Autodesk Inventor part; units mm, degrees
ref_plane "Plan YZ" through (0, 0, 0) normal (1, 0, 0) x (0, 1, 0)
ref_plane "Plan XZ" through (0, 0, 0) normal (0, 1, 0) x (-1, 0, 0)
ref_plane "Plan XY" through (0, 0, 0) normal (0, 0, 1) x (1, 0, 0)
sketch "Esquisse7" plane through (0, 0, 0) normal (0, 0, 1) x (1, 0, 0)
  line L0 (-88, -26) -> (-88, 26)
  line L1 (-88, 26) -> (-83, 26)
  line L2 (-83, 26) -> (-83, 29)
  line L3 (-83, 29) -> (-68, 29)
  line L4 (-68, 29) -> (-68, 26)
  line L5 (-68, 26) -> (-7.5, 26)
  line L6 (-7.5, 26) -> (-7.5, 29)
  line L7 (-7.5, 29) -> (7.5, 29)
  line L8 (7.5, 29) -> (7.5, 26)
  line L9 (7.5, 26) -> (68, 26)
  line L10 (68, 26) -> (68, 29)
  line L11 (68, 29) -> (83, 29)
  line L12 (83, 29) -> (83, 26)
  line L13 (83, 26) -> (88, 26)
  line L14 (88, 26) -> (88, -26)
  line L15 (88, -26) -> (83, -26)
  line L16 (83, -26) -> (83, -29)
  line L17 (83, -29) -> (68, -29)
  line L18 (68, -29) -> (68, -26)
  line L19 (7.5, -26) -> (7.5, -29)
  line L20 (7.5, -26) -> (68, -26)
  line L21 (7.5, -29) -> (-7.5, -29)
  line L22 (-7.5, -29) -> (-7.5, -26)
  line L23 (-7.5, -26) -> (-68, -26)
  line L24 (-68, -26) -> (-68, -29)
  line L25 (-68, -29) -> (-83, -29)
  line L26 (-83, -29) -> (-83, -26)
  line L27 (-83, -26) -> (-88, -26)
  line L28 (0, -40.6) -> (0, 40.6) construction
  line L29 (-123.2, 0) -> (123.2, 0) construction
  dimension "d33" = 52
  dimension "d34" = 15
  dimension "d35" = 3
  dimension "d36" = 5
  dimension "d65" = 176
extrude "Extrusion2" add sketch "Esquisse7" against normal blind 3
sketch "Esquisse8" plane through (0, 0, 0) normal (0, 0, 1) x (1, 0, 0)
  point P0 (0, 0)
  point P1 (7.5, 26)
  point P2 (-7.5, 26)
  point P3 (-83, 26)
  point P4 (-68, 26)
  point P5 (-83, -26)
  point P6 (-68, -26)
  point P7 (-7.5, -26)
  point P8 (7.5, -26)
  point P9 (68, -26)
  point P10 (83, -26)
  point P11 (68, 26)
  point P12 (83, 26)
  point P13 (83, 26)
  point P14 (68, -26)
  point P15 (83, 26)
hole "Perçage2" at (7.5, 26, 0) at (-7.5, 26, 0) at (-83, 26, 0) at (-68, 26, 0) at (-83, -26, 0) at (-68, -26, 0) at (-7.5, -26, 0) at (7.5, -26, 0) at (68, -26, 0) at (83, -26, 0) at (68, 26, 0) at (83, 26, 0) direction (0, 0, -1) diameter 1 end through all
chamfer "Chanfrein3" distance 1 angle 45 12 edges at (-83, -29, -1.5) (-68, -29, -1.5) (-83, 29, -1.5) (-68, 29, -1.5) (-7.5, 29, -1.5) (7.5, 29, -1.5) (68, 29, -1.5) (83, 29, -1.5) (68, -29, -1.5) (83, -29, -1.5) (-7.5, -29, -1.5) (7.5, -29, -1.5)
properties part number "P1704_102" material "Plastique PMMA"
Geometry: final body of the model. Coordinates: model frame, mm. A direction names the side the tool comes from. Coordinates: 2 decimals unless noted, no trailing zeros. Loops run counter-clockwise (first coordinate to the right, second up) from the corner with the lowest first, then second, coordinate; pieces in that order, holes last. Notation, with made-up numbers: (37.5, 52.5) - (43.5, 52.5) arc R11 ccw to (43.5, 62.5) - close; hole circle Ø3 at (-19.5, 76). An arc over 180 degrees is marked (long way). One line per question, with ' | ' between items. Start each with the question number.
(1) Reachability of faces 1 (the flat face through (-86, -26, -1)), 2 (the flat face through (86, -26, -1)), 3 (the flat face through (-86, 26, -1)), 4 (the flat face through (-37, -26, -1)) from +Z, -Z, +X, -X, +Y, -Y: full face, straight path, thin tool, end or side. Return the list, or none.
(2) First-contact query: pin 1 (1.6 mm diameter, centred on y = 27.5, z = -1.5, fed in from -X); pin 2 (0.9 mm diameter, centred on x = -86.5, z = -1, fed in from -Y); pin 3 (0.8 mm diameter, centred on y = 27.5, z = -1, fed in from +X). Flat tips, straight axial feed; report the tip coordinate or a pass-through.
(3) Draft query along X for faces 5 (the flat face through (0, -29, -1)), 6 (the flat face through (-88, 0, -1)), 7 (the flat face through (37, -26, -1)). Return one class per face: +X half, -X half, draft (parallel to the pull), parting line (faces both ways), or undercut.
(4) Ray query, L1, parallel to Y at x = 27, z = -1.65. Return the intervals inside material, ascending. Write a range as from..to.
(5) Cut plane A-A on x = 62. Output: boundary loops of the cut face in (y, z), and give its area (3 significant figures).
Here are the results:
1) face 1: +Z, -Z, -X, -Y | face 2: +Z, -Z, +X, -Y | face 3: +Z, -Z, -X, +Y | face 4: +Z, -Z, -Y
2) pin 1: x = -83 | pin 2: y = -26 | pin 3: x = 83
3) face 5: draft | face 6: -X half | face 7: undercut
4) L1: -26..26
5) outline: (-26, -3) - (26, -3) - (26, 0) - (-26, 0) - close | area: 156 mm²
